```python
from build123d import *

# Parameters (mm, degrees)
ESBO_O1_R                = 8
ESBO_O1_R_2              = 2.5
RESSALTO_EXTRUS_O1_DEPTH = 5
ESBO_O2_R                = 6.8
ESBO_O2_R_2              = 3.7
CORTE_EXTRUS_O1_DEPTH    = 0.5
CORTE_EXTRUS_O2_START    = -0.5
ESBO_O3_R                = 6.8
ESBO_O3_R_2              = 3.7
CORTE_EXTRUS_O2_DEPTH    = 0.5
FILETE1_R                = 0.5


with BuildPart() as part:
    # Esboço1 → Ressalto-extrusão1 (new body)
    with BuildSketch(Plane.XY):
        Circle(ESBO_O1_R)
        Circle(ESBO_O1_R_2, mode=Mode.SUBTRACT)
    extrude(amount=RESSALTO_EXTRUS_O1_DEPTH)

    # Esboço2 → Corte-extrusão1 (cut)
    with BuildSketch(Plane.XY.offset(5)):
        Circle(ESBO_O2_R)
        Circle(ESBO_O2_R_2, mode=Mode.SUBTRACT)
    extrude(amount=-CORTE_EXTRUS_O1_DEPTH, mode=Mode.SUBTRACT)

    # Esboço3 → Corte-extrusão2 (cut)
    with BuildSketch(Plane(origin=(0, 0, 0), x_dir=(-1, 0, 0), z_dir=(0, 0, -1)).offset(CORTE_EXTRUS_O2_START)):
        with Locations(Location((0, 0, 0), (0, 0, 180))):
            Circle(ESBO_O3_R)
        with Locations(Location((0, 0, 0), (0, 0, 180))):
            Circle(ESBO_O3_R_2, mode=Mode.SUBTRACT)
    extrude(amount=CORTE_EXTRUS_O2_DEPTH, mode=Mode.SUBTRACT)

    # Filete1
    filete1_edges = [part.edges().sort_by_distance(p)[0] for p in [
        (-8, 0, 0),
        (-8, 0, 5),
        (-2.5, 0, 0),
        (-2.5, 0, 5),
    ]]
    fillet(filete1_edges, radius=FILETE1_R)


solid = part.part
```
Check sheet for the modelled part. Datum: model origin and axes. Units: mm. A direction names the side the tool comes from. Coordinates: 2 decimals unless noted, no trailing zeros. Loops run counter-clockwise (first coordinate to the right, second up) from the corner with the lowest first, then second, coordinate; pieces in that order, holes last. Notation, with made-up numbers: M 13,5.25 L 24,5.25 A36 ccw 24,40.25 Z; hole C 68.5,-11 d3. An arc over 180 degrees is marked long. Answer as a JSON object with one key per item and string values.
1. Depth check by flat-ended pin: P1, Ø4.5, axis at x = 0, y = 0, coming from the -Z side; P2, Ø3, axis at y = 4.5, z = 0.5, coming from the +X side; P3, Ø3, axis at x = 1, z = 2, coming from the -Y side. Enter the tip coordinate at first touch or a pass-through.
Outcome:
{"P1": "through", "P2": "x = 7.42", "P3": "y = -8"}
2. Access from +Z, -Z, +X, -X, +Y, -Y to the whole of each face (thin tool, end or side, straight path). Record for faces 4 (the flat face through (2, -7, 0)), 5 (the cylindrical face through (-0.802, -3.612, 4.754)), 6 (the cylindrical face through (-1.47, 6.64, 0.25)).
Outcome:
{"face 4": "-Z, +X, -X, +Y, -Y", "face 5": "+Z", "face 6": "-Z"}
3. Scan lines: L1, parallel to Y at x = -0.5, z = 4.8; L2, parallel to Y at x = 0, z = 3; L3, parallel to Y at x = 0, z = 4.6. Record each from-to range of solid material in increasing order. Write a range as from..to.
Outcome:
{"L1": "-7.88..-6.78, -3.67..-2.55, 2.55..3.67, 6.78..7.88", "L2": "-8..-2.5, 2.5..8", "L3": "-7.99..-6.8, -3.7..-2.51, 2.51..3.7, 6.8..7.99"}
4. Sectioned sample at C-C on z = 3.75. Record the cut outline in (x, y).
Outcome:
{"outline": "C 0,0 d16; hole C 0,0 d5"}
5. Release check for a two-part mould opening along X. For faces 1 (the cylindrical face through (-1.73, -7.81, 2.47)), 2 (the cylindrical face through (-0.802, 3.612, 0.254)), 3 (the flat face through (2, -7, 5)) record: pulls with the +X half, pulls with the -X half, needs draft (parallel to the pull), parting line crosses it, or undercut.
Outcome:
{"face 1": "parting line crosses it", "face 2": "undercut", "face 3": "needs draft"}
